Read the model definition and answer for the solid it produces. Units are mm, in the model's axes. Face numbers are marked on the shaded views. A direction names the side the tool comes from. Coordinates: 2 decimals unless noted, no trailing zeros. Write each question's results on one line, items separated by ' | '.
```python
from build123d import *

# Parameters (mm, degrees)
SKETCH1_R           = 13
BOSS_EXTRUDE1_DEPTH = 20
SKETCH2_R           = 4
CUT_EXTRUDE1_DEPTH  = 15
SKETCH3_W           = 12
SKETCH3_H           = 24
BOSS_EXTRUDE2_DEPTH = 70
CHAMFER1_SIZE       = 2
BOSS_EXTRUDE3_DEPTH = 10
CHAMFER2_SIZE       = 2
SKETCH5_W           = 16
SKETCH5_H           = 20
BOSS_EXTRUDE4_DEPTH = 15
CHAMFER3_SIZE       = 2
SKETCH6_R           = 7.5
BOSS_EXTRUDE5_DEPTH = 2
CUT_EXTRUDE2_START  = -20
CUT_EXTRUDE2_DEPTH  = 20
CHAMFER4_SIZE       = 2
SKETCH8_R           = 5
BOSS_EXTRUDE6_DEPTH = 2.5
FILLET1_R           = 1
FILLET2_R           = 1


# Some blends are built 0.0001 mm under size
with BuildPart() as part:
    # Sketch1 → Boss-Extrude1 (new body)
    with BuildSketch(Plane(origin=(0, 0, 0), x_dir=(0, 0, -1), z_dir=(1, 0, 0))):
        Circle(SKETCH1_R)
    extrude(amount=BOSS_EXTRUDE1_DEPTH)

    # Sketch2 → Cut-Extrude1 (cut)
    with BuildSketch(Plane.ZY):
        Circle(SKETCH2_R)
    extrude(amount=-CUT_EXTRUDE1_DEPTH, mode=Mode.SUBTRACT)

    # Sketch3 → Boss-Extrude2 (add)
    with BuildSketch(Plane(origin=(20, 0, 0), x_dir=(0, 0, -1), z_dir=(1, 0, 0))):
        Rectangle(SKETCH3_W, SKETCH3_H)
    extrude(amount=BOSS_EXTRUDE2_DEPTH)

    # Chamfer1
    # the kernel refuses this chamfer: 2 mm, written as the material it takes off along each edge
    with BuildSketch(Plane(origin=(20, -12, -6), x_dir=(0, 0.9996219169112968, -0.027495876610586487), z_dir=(1, 0, 0)), Plane(origin=(20, 12, 6), x_dir=(0, -0.9996219169112968, 0.027495876610586487), z_dir=(1, 0, 0)), Plane(origin=(20, -12, 6), x_dir=(0, -0.027495876610586494, -0.9996219169112968), z_dir=(1, 0, 0))) as chamfer1_piece_1:
        Polygon((CHAMFER1_SIZE * 0.999621916911, CHAMFER1_SIZE * 0.0274958766106), (-CHAMFER1_SIZE * 0.0274958766106, CHAMFER1_SIZE * 0.999621916911), (0, 0), align=None)
    extrude(amount=75.143365976, mode=Mode.SUBTRACT)
    with BuildSketch(Plane(origin=(20, 12, -6), x_dir=(0, -0.9996219169112968, -0.027495876610586487), z_dir=(1, 0, 0))) as chamfer1_piece_2:
        Polygon((CHAMFER1_SIZE * 0.999621916911, -CHAMFER1_SIZE * 0.0274958766106), (-CHAMFER1_SIZE * 0.0274958766106, -CHAMFER1_SIZE * 0.999621916911), (0, 0), align=None)
    extrude(amount=75.143365976, mode=Mode.SUBTRACT)

    # Sketch4 → Boss-Extrude3 (add, symmetric)
    with BuildSketch(Plane.XY):
        Polygon((28, -10), (38, 20), (73, 20), (88, 15), (118, 15), (118, -15), (43, -15), align=None)
    extrude(amount=BOSS_EXTRUDE3_DEPTH, both=True)

    # Chamfer2
    chamfer2_edges = [part.edges().sort_by_distance(p)[0] for p in [
        (80.5, -15, -10),
        (103, 15, -10),
        (55.5, 20, -10),
        (80.5, -15, 10),
        (103, 15, 10),
        (55.5, 20, 10),
    ]]
    chamfer(chamfer2_edges, length=CHAMFER2_SIZE)

    # Sketch5 → Boss-Extrude4 (add)
    with BuildSketch(Plane(origin=(118, 0, 0), x_dir=(0, 0, -1), z_dir=(1, 0, 0))):
        Rectangle(SKETCH5_W, SKETCH5_H)
    extrude(amount=BOSS_EXTRUDE4_DEPTH)

    # Chamfer3
    chamfer3_edges = [part.edges().sort_by_distance(p)[0] for p in [
        (125.5, -10, -8),
        (125.5, 10, -8),
        (125.5, 10, 8),
        (125.5, -10, 8),
    ]]
    chamfer(chamfer3_edges, length=CHAMFER3_SIZE)

    # Sketch6 → Boss-Extrude5 (add)
    with BuildSketch(Plane(origin=(133, 0, 0), x_dir=(0, 0, -1), z_dir=(1, 0, 0))):
        with Locations(Location((0, 0, 0), (0, 0, 90))):
            Circle(SKETCH6_R)
    extrude(amount=BOSS_EXTRUDE5_DEPTH)

    # Sketch7 → Cut-Extrude2 (cut)
    with BuildSketch(Plane(origin=(135, 0, 0), x_dir=(0, 0, -1), z_dir=(1, 0, 0)).offset(CUT_EXTRUDE2_START)):
        with BuildLine():
            Line((5, -0.75), (5, 0.75))
            Line((5, 0.75), (3.929058411, 0.75))
            ThreePointArc((3.929058411, 0.75), (2.828427125, 2.828427125), (0.75, 3.929058411))
            Line((0.75, 3.929058411), (0.75, 5))
            Line((0.75, 5), (-0.75, 5))
            Line((-0.75, 5), (-0.75, 3.929058411))
            ThreePointArc((-0.75, 3.929058411), (-2.828427125, 2.828427125), (-3.929058411, 0.75))
            Line((-3.929058411, 0.75), (-5, 0.75))
            Line((-5, 0.75), (-5, -0.75))
            Line((-5, -0.75), (-3.929058411, -0.75))
            ThreePointArc((-3.929058411, -0.75), (-2.828427125, -2.828427125), (-0.75, -3.929058411))
            Line((-0.75, -3.929058411), (-0.75, -5))
            Line((-0.75, -5), (0.75, -5))
            Line((0.75, -5), (0.75, -3.929058411))
            ThreePointArc((0.75, -3.929058411), (2.828427125, -2.828427125), (3.929058411, -0.75))
            Line((3.929058411, -0.75), (5, -0.75))
        make_face()
    extrude(amount=CUT_EXTRUDE2_DEPTH, mode=Mode.SUBTRACT)

    # Chamfer4
    chamfer4_edges = [part.edges().sort_by_distance(p)[0] for p in [
        (135, -7.5, 0),
    ]]
    chamfer(chamfer4_edges, length=CHAMFER4_SIZE - 0.0001)  # a hair under: the kernel refuses the full size

    # Sketch8 → Boss-Extrude6 (add, symmetric)
    with BuildSketch(Plane.XY):
        with BuildLine():
            Line((118, -15), (84, -15))
            Line((84, -15), (84, -30))
            ThreePointArc((84, -30), (89, -38.660254038), (99, -38.660254038))
            Line((99, -38.660254038), (115, -29.422649731))
            ThreePointArc((115, -29.422649731), (117.196152423, -27.226497308), (118, -24.226497308))
            Line((118, -24.226497308), (118, -15))
        make_face()
        with Locations((94, -30)):
            Circle(SKETCH8_R, mode=Mode.SUBTRACT)
    extrude(amount=BOSS_EXTRUDE6_DEPTH, both=True)

    # Fillet1
    fillet1_edges = [part.edges().sort_by_distance(p)[0] for p in [
        (0, 0, 13),
    ]]
    fillet(fillet1_edges, radius=FILLET1_R)

    # Fillet2
    fillet2_edges = [part.edges().sort_by_distance(p)[0] for p in [
        (107, -34.041451884, -2.5),
        (117.196152423, -27.226497308, -2.5),
        (118, -19.613248654, 2.5),
        (84, -22.5, -2.5),
        (89, -38.660254038, -2.5),
        (107, -34.041451884, 2.5),
        (117.196152423, -27.226497308, 2.5),
        (84, -22.5, 2.5),
        (89, -38.660254038, 2.5),
        (118, -19.613248654, -2.5),
    ]]
    fillet(fillet2_edges, radius=FILLET2_R)


solid = part.part
```
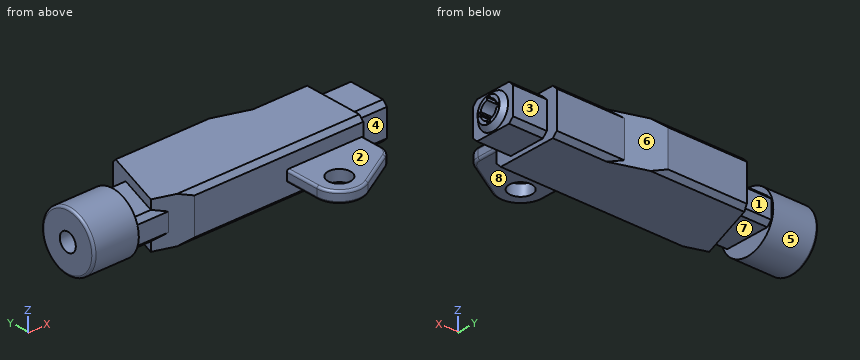
(1) Given pin 1 (12 mm diameter, centred on x = 107.5, y = -30.5, fed in from -Z); pin 2 (0.5 mm diameter, centred on x = 120.5, y = -4.5, fed in from -Z); pin 3 (6.5 mm diameter, centred on y = -0.5, z = 0, fed in from -X); pin 4 (4 mm diameter, centred on x = 54, y = -18.5, fed in from +Z), each flat-ended and moving along its own axis, determine where each tip first touches the part or whether it passes through.
Conclusion:
pin 1: z = -2.5 | pin 2: z = -8 | pin 3: x = 15 | pin 4: through
(2) For the marked faces 1, 2, 3, 4 and 5, determine the directions among +Z, -Z, +X, -X, +Y, -Y from which every point of the face is accessible in a straight line to the end or side of a thin tool.
Conclusion:
face 1: +Z, -Z, +Y | face 2: +Z, +X, -X, -Y | face 3: +Z, -Z, +X, +Y | face 4: +Z, -Z, +X, -Y | face 5: -X
(3) Straight lines are drawn through the part: line 1 (X direction, y = -3.5, z = 0.25); line 2 (Y direction, x = 58, z = -1.5); line 3 (Y direction, x = 6, z = 0). For each, find the intervals that lie inside material, in ascending order.
Conclusion:
line 1: 15 to 115 | line 2: -15 to 20 | line 3: -13 to -4, 4 to 13
(4) The mould has two halves that part along X. Classify the marked faces 6, 7 and 8: pulls with the +X half, pulls with the -X half, needs draft (parallel to the pull), parting line crosses it, or undercut.
Conclusion:
face 6: pulls with the +X half | face 7: undercut | face 8: needs draft
